Could you check a few things on this model? Use its own coordinates, in mm. Face numbers are marked on the shaded views. A direction names the side the tool comes from. Give positions to 0.01 mm unless a question says otherwise; leave off trailing zeros. Write each loop counter-clockwise with the first axis right and the second up, starting at its lowest first coordinate (ties: lowest second). Pieces come first, ordered by that corner, then holes. Notation, with made-up numbers: (-5.75, -2) - (2.25, -2) arc R13 cw to (2.25, 10) - close; hole circle Ø2 at (51, 41.25). An arc over 180 degrees is marked (long way). Answer as a JSON object with one key per item and string values. Group by question number.
```python
from build123d import *

# Parameters (mm, degrees)
F0_R      = 8.5
F1_DEPTH  = 8
F3_DEPTH  = 4
F4_R      = 7.75
F5_DEPTH  = 1.5
F7_R      = 4.5
F8_DEPTH  = 25
F6_R      = 4.5
F9_DEPTH  = 2
F10_R     = 4
F11_DEPTH = 10


with BuildPart() as f1:
    # F0 (on Right) → F1 (new body)
    with BuildSketch(Plane.YZ):
        with Locations((-38.9976724982, 9.3536879867)):
            Circle(F0_R)
    extrude(amount=F1_DEPTH)

    # F2 (on face) → F3 (cut)
    with BuildSketch(Plane.YZ.offset(8)):
        Polygon((-34.8214355244, 16.4690979189), (-43.0716797709, 16.5281202644), (-47.2479167448, 9.4127103322), (-43.1739094721, 2.2382780545), (-34.9236652255, 2.1792557091), (-30.7474282517, 9.2946656413), align=None)
    extrude(amount=-F3_DEPTH, mode=Mode.SUBTRACT)

    # F4 (on face) → F5 (cut)
    with BuildSketch(Plane(origin=(0, 0, 0), x_dir=(0, -1, 0), z_dir=(-1, 0, 0))):
        with Locations((38.9976724982, 9.3536879867)):
            Circle(F4_R)
    extrude(amount=-F5_DEPTH, mode=Mode.SUBTRACT)

    # F7 (on face) → F8 (cut)
    with BuildSketch(Plane.YZ.offset(4)):
        with Locations((-38.9976724982, 9.3536879867)):
            Circle(F7_R)
    extrude(amount=-F8_DEPTH, mode=Mode.SUBTRACT)

    # F6 (on face) → F9 (join)
    with BuildSketch(Plane(origin=(0, 0, 0), x_dir=(0, -1, 0), z_dir=(-1, 0, 0))):
        with Locations((38.9976724982, 9.3536879867)):
            Circle(F6_R)
    extrude(amount=-F9_DEPTH)

    # F10 (on face) → F11 (cut)
    with BuildSketch(Plane(origin=(0, 0, 0), x_dir=(0, -1, 0), z_dir=(-1, 0, 0))):
        with Locations((38.9976724982, 9.3536879867)):
            Circle(F10_R)
    extrude(amount=-F11_DEPTH, mode=Mode.SUBTRACT)


solid = f1.part
```
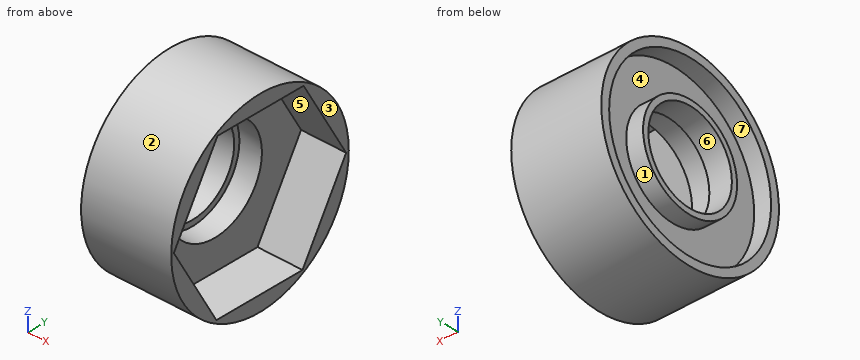
(1) If we mould it in two halves opening along Y, with no side actions, what happens to the marked faces 1, 2, 3 and 4? For each: +Y half, -Y half, draft (parallel to the pull), parting line (faces both ways), or undercut.
(2) Will these pins go through, and if not, where does the flat tip stop? P1, Ø2.5, axis at y = -37.5, z = 8, coming from the +X side; P2, Ø1, axis at x = 1, y = -42.5, coming from the -Z side; P3, Ø1, axis at y = -33.5, z = 13, coming from the -X side; P4, Ø1, axis at x = 4, z = 14, coming from the +Y side.
(3) I need wall thicknesses on L1, parallel to Z at x = 0.5, y = -39.25; L2, parallel to X at y = -40.5, z = 13.5; L3, parallel to X at y = -35.75, z = 15.5. Which ranges of each line are inside material? Lowest first, please.
(4) I want a section at B-B, the plane z = 7.5. Please give me the cut outline in (x, y).
(5) For the marked faces 5, 6 and 7, which set-ups out of +Z, -Z, +X, -X, +Y, -Y let a thin tool reach every point of the face, with its end or its side?
(6) I want a section at D-D, the plane z = 4.5. Please give me the cut outline in (x, y), and give its area (3 significant figures).
(7) I want a section at C-C, the plane x = 7.5. Please give me the cut outline in (y, z), and give its area (3 significant figures).
(8) I want a section at A-A, the plane y = -40.75. Please give me the cut outline in (x, z).
Entries:
{
 "1": {"face 1": "undercut", "face 2": "parting line", "face 3": "draft", "face 4": "undercut"},
 "2": {"P1": "through", "P2": "z = 1.4", "P3": "x = 1.5", "P4": "y = -31.58"},
 "3": {"L1": "0.86 to 1.61, 4.86 to 5.36, 13.35 to 13.85, 17.1 to 17.85", "L2": "0 to 2", "L3": "1.5 to 4"},
 "4": {"outline": "(0, -47.29) - (8, -47.29) - (8, -46.16) - (4, -46.16) - (4, -43.1) - (2, -43.1) - (2, -42.54) - (0, -42.54) - (0, -43.1) - (1.5, -43.1) - (1.5, -46.52) - (0, -46.52) - close; (0, -35.45) - (2, -35.45) - (2, -34.9) - (4, -34.9) - (4, -31.8) - (8, -31.8) - (8, -30.7) - (0, -30.7) - (0, -31.47) - (1.5, -31.47) - (1.5, -34.9) - (0, -34.9) - close"},
 "5": {"face 5": "+X", "face 6": "+X, -X", "face 7": "-X"},
 "6": {"outline": "(0, -45.98) - (8, -45.98) - (8, -44.46) - (4, -44.46) - (4, -33.56) - (8, -33.56) - (8, -32.02) - (0, -32.02) - (0, -32.96) - (1.5, -32.96) - (1.5, -45.04) - (0, -45.04) - close", "area": "49.9 mm^2"},
 "7": {"outline": "circle Ø17 at (-39, 9.35); hole (-47.25, 9.41) - (-43.17, 2.24) - (-34.92, 2.18) - (-30.75, 9.29) - (-34.82, 16.47) - (-43.07, 16.53) - close", "area": "50.1 mm^2"},
 "8": {"outline": "(0, 1.04) - (8, 1.04) - (8, 2.22) - (4, 2.22) - (4, 5.21) - (2, 5.21) - (2, 5.76) - (0, 5.76) - (0, 5.21) - (1.5, 5.21) - (1.5, 1.8) - (0, 1.8) - close; (0, 12.95) - (2, 12.95) - (2, 13.5) - (4, 13.5) - (4, 16.51) - (8, 16.51) - (8, 17.67) - (0, 17.67) - (0, 16.9) - (1.5, 16.9) - (1.5, 13.5) - (0, 13.5) - close"}
}
